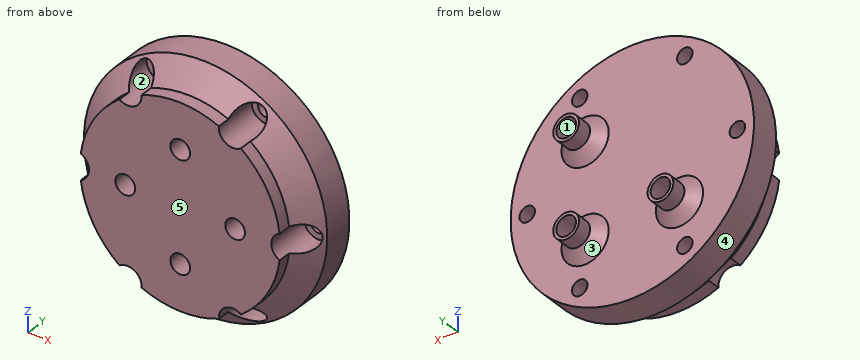
```python
from build123d import *

# Parameters (mm, degrees)
CBORE_FOR_M3_HEX_SOCKET_HEAD_CAP_SCREW1_D           = 3.6
CBORE_FOR_M3_HEX_SOCKET_HEAD_CAP_SCREW1_CBORE_D     = 6.5
CBORE_FOR_M3_HEX_SOCKET_HEAD_CAP_SCREW1_CBORE_DEPTH = 10.4
HOLEWZD2_D                                          = 4.6
HOLEWZD2_DEPTH                                      = 7
HOLEWZD2_TIP                                        = 2.3
SKETCH9_R                                           = 3
BOSS_EXTRUDE1_DEPTH                                 = 6
HOLEWZD1_D                                          = 4.6
HOLEWZD1_DEPTH                                      = 7
CHAMFER1_SIZE                                       = 2.5


with BuildPart() as part:
    # Sketch3 → Revolve1 (revolve)
    with BuildSketch(Plane.XY, mode=Mode.PRIVATE) as revolve1_sk:
        Polygon((0, 0), (23.365, 0), (23.365, 3), (28.365, 8), (28.365, 15), (0, 15), align=None)
    revolve(revolve1_sk.sketch.rotate(Axis((0, 0, 0), (0, 1, 0)), 90), axis=Axis((0, 0, 0), (0, 1, 0)))

    # CBORE for M3 Hex Socket Head Cap Screw1 (through all)
    with Locations(Plane(origin=(0, 0, 0), x_dir=(-1, 0, 0), z_dir=(0, -1, 0))):
        with Locations((-24.5, 0), (12.25, 21.217622393), (-12.25, 21.217622393), (-12.25, -21.217622393), (12.25, -21.217622393), (24.5, 0)):
            CounterBoreHole(CBORE_FOR_M3_HEX_SOCKET_HEAD_CAP_SCREW1_D / 2, CBORE_FOR_M3_HEX_SOCKET_HEAD_CAP_SCREW1_CBORE_D / 2, CBORE_FOR_M3_HEX_SOCKET_HEAD_CAP_SCREW1_CBORE_DEPTH)

    # HoleWzd2
    with Locations(Plane(origin=(0, 0, 0), x_dir=(-1, 0, 0), z_dir=(0, -1, 0))):
        with Locations((-12.8, 0), (0, 12.8), (12.8, 0), (0, -12.8)):
            Hole(HOLEWZD2_D / 2, depth=HOLEWZD2_DEPTH)
            with Locations((0, 0, -(HOLEWZD2_DEPTH + HOLEWZD2_TIP / 2))):  # 90° drill point
                Cone(0, HOLEWZD2_D / 2, HOLEWZD2_TIP, mode=Mode.SUBTRACT)

    # Sketch9 → Boss-Extrude1 (add)
    with BuildSketch(Plane(origin=(0, 15, 0), x_dir=(1, 0, 0), z_dir=(0, 1, 0))):
        with Locations(Location((-11, 11, 0), (0, 0, 270))):
            Circle(SKETCH9_R)
        with Locations(Location((11, 11, 0), (0, 0, 270))):
            Circle(SKETCH9_R)
        with Locations(Location((11, -11, 0), (0, 0, 270))):
            Circle(SKETCH9_R)
    extrude(amount=BOSS_EXTRUDE1_DEPTH)

    # HoleWzd1
    with Locations(Plane(origin=(0, 21, 0), x_dir=(1, 0, 0), z_dir=(0, 1, 0))):
        with Locations((11, -11), (11, 11), (-11, 11)):
            Hole(HOLEWZD1_D / 2, depth=HOLEWZD1_DEPTH)

    # Chamfer1
    chamfer1_edges = [part.edges().sort_by_distance(p)[0] for p in [
        (-11, 15, -14),
        (11, 15, -14),
        (11, 15, 8),
    ]]
    chamfer(chamfer1_edges, length=CHAMFER1_SIZE)


solid = part.part
```
Check sheet for the modelled part. Datum: model origin and axes. Units: mm. Face numbers are marked on the shaded views. A direction names the side the tool comes from. Coordinates: 2 decimals unless noted, no trailing zeros. Loops run counter-clockwise (first coordinate to the right, second up) from the corner with the lowest first, then second, coordinate; pieces in that order, holes last.
1) Sectioned sample at B-B (y = 16.5). Record the boundary of the cut face in (x, z), and give its area (3 significant figures).
2) Gauge pin test, flat ends, axial feed: pin 1 (8 mm diameter, centred on x = -0.5, z = -17.5, fed in from +Y); pin 2 (5 mm diameter, centred on y = 4, z = -19, fed in from -X); pin 3 (7.5 mm diameter, centred on x = 0, z = -12.8, fed in from -Y); pin 4 (10 mm diameter, centred on x = -14, y = 18, fed in from +Z). Record the tip position at first contact, or that the pin passes through.
3) Access from +Z, -Z, +X, -X, +Y, -Y to the whole of each face (thin tool, end or side, straight path). Record for the marked faces 1 and 2.
4) Sectioned sample at C-C (y = 11.5). Record the boundary of the cut face in (x, z) (3 decimals), and give its area (3 significant figures).
5) Sectioned sample at A-A (y = 2). Record the boundary of the cut face in (x, z) (3 decimals).
6) Release check for a two-part mould opening along X. For the marked faces 3, 4 and 5 record: released by +X, released by -X, zero draft, split by the parting line, or undercut.
7) Material ranges on probe 1 along Z at (x, y) = (0, 2) (3 decimals); probe 2 along Z at (x, y) = (11, 15.5); probe 3 along X at (y, z) = (11.25, -21), recorded low to high.
Check sheet entries:
1. outline: circle Ø8 at (-11, -11); circle Ø8 at (11, -11); circle Ø8 at (11, 11); hole circle Ø4.6 at (-11, -11); hole circle Ø4.6 at (11, -11); hole circle Ø4.6 at (11, 11)
1. area: 101 mm2
2. pin 1: stops at y = 15
2. pin 2: stops at x = -19.73
2. pin 3: stops at y = 0
2. pin 4: stops at z = 26.54
3. face 1: +Y
3. face 2: -Y
4. outline: circle Ø56.73 at (0, 0); hole circle Ø3.6 at (-24.5, 0); hole circle Ø3.6 at (-12.25, -21.218); hole circle Ø3.6 at (-12.25, 21.218); hole circle Ø3.6 at (12.25, -21.218); hole circle Ø3.6 at (12.25, 21.218); hole circle Ø3.6 at (24.5, 0)
4. area: 2,470 mm2
5. outline: (-23.176, -2.968) arc R23.365 ccw to (-14.158, -18.587) arc R3.25 cw to (-9.018, -21.555) arc R23.365 ccw to (9.018, -21.555) arc R3.25 cw to (14.158, -18.587) arc R23.365 ccw to (23.176, -2.968) arc R3.25 cw to (23.176, 2.968) arc R23.365 ccw to (14.158, 18.587) arc R3.25 cw to (9.018, 21.555) arc R23.365 ccw to (-9.018, 21.555) arc R3.25 cw to (-14.158, 18.587) arc R23.365 ccw to (-23.176, 2.968) arc R3.25 cw to start; hole circle Ø4.6 at (-12.8, 0); hole circle Ø4.6 at (0, -12.8); hole circle Ø4.6 at (0, 12.8); hole circle Ø4.6 at (12.8, 0)
6. face 3: undercut
6. face 4: split by the parting line
6. face 5: zero draft
7. probe 1: z = -23.365 to -15.1, -10.5 to 10.5, 15.1 to 23.365
7. probe 2: z = -16 to -13.3, -8.7 to -6, 6 to 8.7, 13.3 to 16
7. probe 3: x = -19.07 to -14.04, -10.46 to 10.46, 14.04 to 19.07
